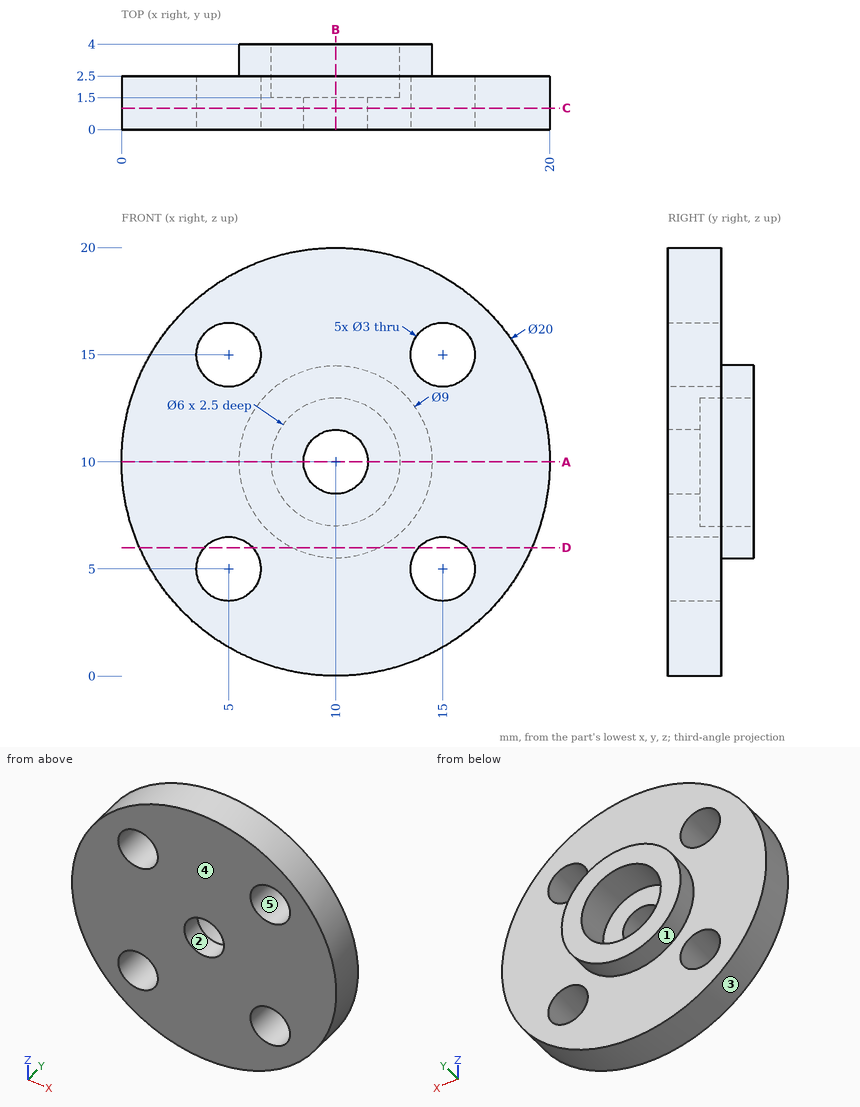
Job drawing, mm, ordinate dimensions from the low corner. One solid piece. A direction names the side the tool comes from. Coordinates: 2 decimals unless noted, no trailing zeros. Order: outer loops, then holes, each group sorted by start corner. A loop starts at its lowest first (then second) coordinate and runs counter-clockwise, first axis right, second up. Notation, with made-up numbers: M -19,60.25 L 13,60.25 A10 ccw 13,78.25 Z; hole C 11.25,49 d9. An arc over 180 degrees is marked long. One line per question, with ' | ' between items.
Q1. Two-plate mould, pull along X, no slides. Class the marked faces 3, 4 and 5: +X half, -X half, draft (parallel to the pull), parting line (faces both ways), or undercut.
A:
face 3: parting line | face 4: draft | face 5: undercut
Q2. Slice it at A-A (z = 10). Give the cut face in (x, y), and give its area (3 significant figures).
A:
outline: M 0,0 L 8.5,0 L 8.5,1.5 L 7,1.5 L 7,4 L 5.5,4 L 5.5,2.5 L 0,2.5 Z; M 11.5,0 L 20,0 L 20,2.5 L 14.5,2.5 L 14.5,4 L 13,4 L 13,1.5 L 11.5,1.5 Z | area: 44.0 mm^2
Q3. 3-axis set-ups, long thin cutter, end or side, ignore diameter. For the marked faces 1 and 2: which of +Z, -Z, +X, -X, +Y, -Y reach the whole face in a straight line?
A:
face 1: +Y | face 2: +Y, -Y
Q4. Slice it at D-D (z = 6). Give the cut face in (x, y), and give its area (3 significant figures).
A:
outline: M 0.83,0 L 3.88,0 L 3.88,2.5 L 0.83,2.5 Z; M 6.12,0 L 13.88,0 L 13.88,2.5 L 12.06,2.5 L 12.06,4 L 7.94,4 L 7.94,2.5 L 6.12,2.5 Z; M 16.12,0 L 19.17,0 L 19.17,2.5 L 16.12,2.5 Z | area: 40.8 mm^2
Q5. Slice it at B-B (x = 10). Give the cut face in (y, z).
A:
outline: M 0,0 L 2.5,0 L 2.5,5.5 L 4,5.5 L 4,7 L 1.5,7 L 1.5,8.5 L 0,8.5 Z; M 0,11.5 L 1.5,11.5 L 1.5,13 L 4,13 L 4,14.5 L 2.5,14.5 L 2.5,20 L 0,20 Z
Q6. Slice it at C-C (y = 1). Give the cut face in (x, z).
A:
outline: C 10,10 d20; hole C 5,5 d3; hole C 5,15 d3; hole C 10,10 d3; hole C 15,5 d3; hole C 15,15 d3
Q7. Pin check, flat tips, straight feed: P1, Ø3, axis at x = 10.5, z = 10.5, coming from the +Y side; P2, Ø1.5, axis at x = 6.5, z = 5.5, coming from the +Y side; P3, Ø1, axis at y = 2, z = 6.5, coming from the -X side. Stop position of each tip, or through.
A:
P1: stops at y = 1.5 | P2: stops at y = 2.5 | P3: stops at x = 0.46
Q8. Drill centre lines: line 1 (X direction, y = 0.6, z = 10); line 2 (X direction, y = 0.5, z = 5); line 3 (X direction, y = 1.25, z = 4.75). Where is each one in solid material? Low to high.
A:
line 1: x = 0 to 8.5, 11.5 to 20 | line 2: x = 1.34 to 3.5, 6.5 to 13.5, 16.5 to 18.66 | line 3: x = 1.49 to 3.52, 6.48 to 13.52, 16.48 to 18.51
